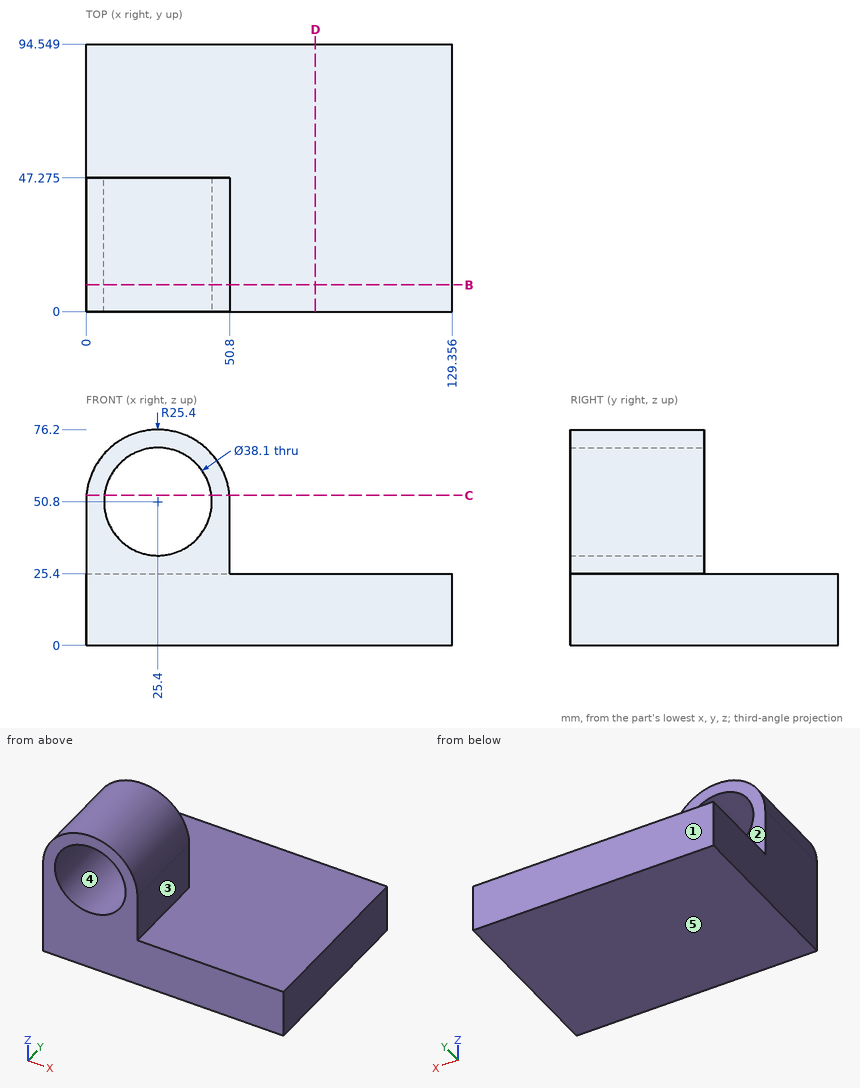
Geometry check sheet. Reference: drawing and pictorial views, mm from the part's lowest x, y, z. A direction names the side the tool comes from. Round coordinates to 2 decimals unless told otherwise and drop trailing zeros. Order: outer loops, then holes, each group sorted by start corner. A loop starts at its lowest first (then second) coordinate and runs counter-clockwise, first axis right, second up. Notation, with made-up numbers: (-25.5, 68.25) - (26.5, 68.25) arc R29 ccw to (26.5, 106.25) - close; hole circle Ø11 at (3.25, 72). An arc over 180 degrees is marked (long way). Use a Markdown table: item, result. Add a question column.
1) Gauge pin test, flat ends, axial feed: P1, Ø3, axis at x = 110.5, z = 15.5, coming from the -Y side; P2, Ø10, axis at y = 19.5, z = 59.5, coming from the -X side; P3, Ø2, axis at x = 106, y = 12.5, coming from the +Z side; P4, Ø1.5, axis at y = 37, z = 66.5, coming from the +X side (1 decimal). Record the tip position at first contact, or that the pin passes through.
2) Mould release check, pull along X, two halves, no side actions. Record for the marked faces 3, 4 and 5: released by +X, released by -X, zero draft, split by the parting line, or undercut.
3) Set-up check for the marked faces 1 and 2: record each of +Z, -Z, +X, -X, +Y, -Y from which the full face is reachable in a straight line by a thin tool's end or side.
4) Section check D-D (x = 81). Record the cut outline in (y, z).
5) Section check B-B (y = 9.5). Record the cut outline in (x, z).
6) Section check C-C (z = 53). Record the cut outline in (x, y) (1 decimal).
7) Thickness scan on line 1 along Z through (x, y) = (25, 28) (1 decimal); line 2 along X through (y, z) = (21, 50); line 3 along Z through (x, y) = (19, 56). Record the ranges inside material, lowest first.
Established:
| question | item | result |
|---|---|---|
| 1 | P1 | y = 0 |
| 1 | P2 | x = 0.27 |
| 1 | P3 | z = 25.4 |
| 1 | P4 | x = 45.9 |
| 2 | face 3 | released by +X |
| 2 | face 4 | undercut |
| 2 | face 5 | zero draft |
| 3 | face 1 | +Z, -Z, +X, -X, +Y |
| 3 | face 2 | +Z, +X, -X, +Y |
| 4 | outline | (0, 0) - (94.55, 0) - (94.55, 25.4) - (0, 25.4) - close |
| 5 | outline | (0, 0) - (129.36, 0) - (129.36, 25.4) - (50.8, 25.4) - (50.8, 50.8) arc R25.4 ccw to (0, 50.8) - close; hole circle Ø38.1 at (25.4, 50.8) |
| 6 | outline | (0.1, 0) - (6.5, 0) - (6.5, 47.3) - (0.1, 47.3) - close; (44.3, 0) - (50.7, 0) - (50.7, 47.3) - (44.3, 47.3) - close |
| 7 | line 1 | 0 to 31.8, 69.8 to 76.2 |
| 7 | line 2 | 0 to 6.37, 44.43 to 50.8 |
| 7 | line 3 | 0 to 25.4 |
